Here's how the part is built. I have some questions about the finished solid (model axes, mm). A direction names the side the tool comes from. Round coordinates to 2 decimals unless told otherwise and drop trailing zeros. Write each loop counter-clockwise with the first axis right and the second up, starting at its lowest first coordinate (ties: lowest second). Pieces come first, ordered by that corner, then holes. Notation, with made-up numbers: M 3.5,-17.5 L 15.5,-17.5 A17 cw 15.5,-7.5 Z; hole C -16.5,11.25 d1. An arc over 180 degrees is marked long. Write item = value, one per line. Start each with the question number.
(1) I want a section at A-A (z = -67). List the corners of the cut face in (x, y) for me.
(2) On a 3-axis mill with a long thin cutter (end or side, diameter ignored), from which of +Z, -Z, +X, -X, +Y, -Y can I reach the whole of each face in a straight line? I mean faces 1 (the cylindrical face through (-13.595, 11.07, -7.855)), 2 (the flat face through (-4, 0, -38.804)), 3 (the flat face through (-4, 6, -71)). Say none if no direction works.
(3) If we mould it in two halves opening along Y, with no side actions, what happens to faces 4 (the flat face through (-6, 6, -19)), 5 (the cylindrical face through (-3.898, 0.132, -52.806)), 6 (the flat face through (-6, -16, -31)), 7 (the cylindrical face through (-13.595, -10.93, -7.855))? For each: released by +Y, released by -Y, zero draft, split by the parting line, or undercut.
(4) I want a section at D-D (x = -15.75). List the corners of the cut face in (y, z) for me, and give its area (3 significant figures).
(5) Will these pins go through, and if not, where does the flat tip stop? pin 1 Ø6 at (x, y) = (-4, -2) entering from +Z; pin 2 Ø4 at (y, z) = (-11, -46.5) entering from -X; pin 3 Ø1 at (x, y) = (-13, 12) entering from -Z; pin 4 Ø9.5 at (x, z) = (-12.81, -13.8) entering from -Y.
(6) I want a section at B-B (y = 0). List the corners of the cut face in (x, z) for me, and give its area (3 significant figures).
(7) I need wall thicknesses on line 1 along Y through (x, z) = (-13.5, -22); line 2 along Z through (x, y) = (-13.25, -13); line 3 along X through (y, z) = (-11, -59). Which ranges of each line are inside material? Lowest first, please.
```python
from build123d import *

# Parameters (mm, degrees)
F0_R     = 6
F1_DEPTH = 16
F3_W     = 12
F3_H     = 25
F3_H_2   = 40
F4_DEPTH = 32.187343


with BuildPart() as f1:
    # F0 (on Front) → F1 (new body, symmetric)
    with BuildSketch(Plane.XZ):
        with BuildLine():
            Line((2.186343, -99.804071), (2.186343, -13.804071))
            ThreePointArc((2.186343, -13.804071), (-24.432607, -4.317238), (-9.813657, -28.501009))
            Line((-9.813657, -28.501009), (-9.813657, -99.804071))
            Line((-9.813657, -99.804071), (2.186343, -99.804071))
        make_face()
        with Locations((-12.813657, -13.804071)):
            Circle(F0_R, mode=Mode.SUBTRACT)
    extrude(amount=F1_DEPTH, both=True)

    # F3 (on offset) → F4 (cut, through all)
    with BuildSketch(Plane.YZ.offset(-30)):
        with BuildLine():
            ThreePointArc((16, -83.804071), (0, -99.461515), (-16, -83.804071))
            Line((-16, -83.804071), (-16, -99.804071))
            Line((-16, -99.804071), (16, -99.804071))
            Line((16, -99.804071), (16, -83.804071))
        make_face()
        with BuildLine():
            Line((-6, -58.804071), (6, -58.804071))
            ThreePointArc((6, -58.804071), (0, -52.804071), (-6, -58.804071))
        make_face()
        with BuildLine():
            ThreePointArc((-6, -83.804071), (0, -89.804071), (6, -83.804071))
            Line((6, -83.804071), (-6, -83.804071))
        make_face()
        with Locations((0, -71.304071)):
            Rectangle(F3_W, F3_H)
        with Locations((0, -18.804071)):
            Rectangle(F3_W, F3_H_2)
    extrude(amount=F4_DEPTH, mode=Mode.SUBTRACT)


solid = f1.part
```
Returned:
q1.outline = M -9.81,-16 L 2.19,-16 L 2.19,-6 L -9.81,-6 Z; M -9.81,6 L 2.19,6 L 2.19,16 L -9.81,16 Z
q2.face_1 = +Y, -Y
q2.face_2 = +Z, +X, -X
q2.face_3 = +X, -X
q3.face_4 = undercut
q3.face_5 = undercut
q3.face_6 = released by -Y
q3.face_7 = zero draft
q4.outline = M -16,-28.51 L -6,-28.51 L -6,-19.04 L -16,-19.04 Z; M -16,-8.57 L -6,-8.57 L -6,0.91 L -16,0.91 Z; M 6,-28.51 L 16,-28.51 L 16,-19.04 L 6,-19.04 Z; M 6,-8.57 L 16,-8.57 L 16,0.91 L 6,0.91 Z
q4.area = 379 mm²
q5.pin_1 = -38.8
q5.pin_2 = -9.81
q5.pin_3 = -28.8
q5.pin_4 = through
q6.outline = M -9.81,-99.46 L 2.19,-99.46 L 2.19,-89.8 L -9.81,-89.8 Z; M -9.81,-52.8 L 2.19,-52.8 L 2.19,-38.8 L -9.81,-38.8 Z
q6.area = 284 mm²
q7.line_1 = -16 to -6, 6 to 16
q7.line_2 = -28.8 to -19.79, -7.82 to 1.19
q7.line_3 = -9.81 to 2.19
